Build history of the part. All positions in model axes, mm. Give positions to 0.01 mm unless a question says otherwise; leave off trailing zeros. Write each loop counter-clockwise with the first axis right and the second up, starting at its lowest first coordinate (ties: lowest second). Pieces come first, ordered by that corner, then holes.
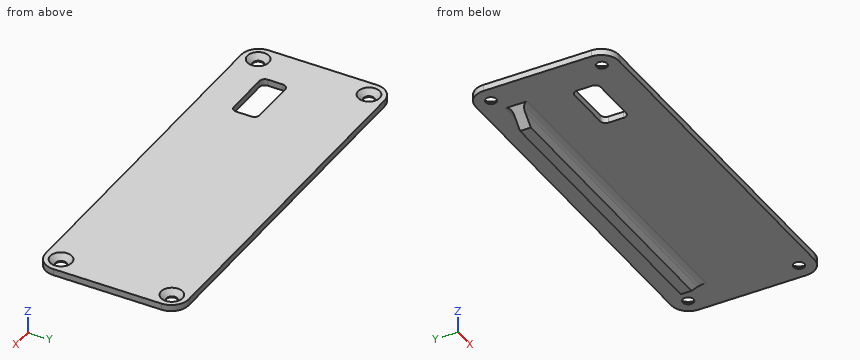
Autodesk Inventor part; units mm, degrees
ref_plane "YZ Plane" through (0, 0, 0) normal (1, 0, 0) x (0, 1, 0)
ref_plane "XZ Plane" through (0, 0, 0) normal (0, 1, 0) x (-1, 0, 0)
ref_plane "XY Plane" through (0, 0, 0) normal (0, 0, 1) x (1, 0, 0)
sketch "Sketch1" plane through (0, 0, 0) normal (0, 0, 1) x (1, 0, 0)
  line L0 (-35.5, 13.25) -> (35.5, 13.25)
  line L1 (35.5, 13.25) -> (35.5, -13.25)
  line L2 (35.5, -13.25) -> (-35.5, -13.25)
  line L3 (-35.5, -13.25) -> (-35.5, 13.25)
  point P0 (0, 0)
  dimension "d0" = 26.5
  dimension "d1" = 71
  dimension "d2" = 35.5
  dimension "d3" = 13.25
extrude "Extrusion1" add sketch "Sketch1" along normal blind 1.2
fillet "Fillet1" radius 3.25 4 edges at (-35.5, 13.25, 0.6) (-35.5, -13.25, 0.6) (35.5, -13.25, 0.6) (35.5, 13.25, 0.6)
sketch "Sketch2" plane through (0, 0, 1.2) normal (0, 0, 1) x (1, 0, 0)
  line L0 (32.25, 13.25) -> (-32.25, 13.25)
  line L1 (-35.5, 10) -> (-35.5, -10)
  line L2 (-32.25, -13.25) -> (32.25, -13.25)
  line L3 (35.5, -10) -> (35.5, 10)
  point P0 (0, 0)
  point P1 (-32.5, 10.25)
  point P2 (32.5, 10.25)
  point P3 (32.5, -10.25)
  point P4 (-32.5, -10.25)
  dimension "d7" = 3
  dimension "d8" = 3
  dimension "d9" = 3
  dimension "d10" = 3
  dimension "d11" = 3
  dimension "d12" = 3
  dimension "d13" = 3
  dimension "d14" = 3
hole "Hole1" at (-32.5, 10.25, 1.2) at (32.5, 10.25, 1.2) at (32.5, -10.25, 1.2) at (-32.5, -10.25, 1.2) direction (0, 0, -1) diameter 2 depth 4 tip angle 118 countersink diameter 4 countersink angle 90
sketch "Sketch3" plane through (0, 0, 1.2) normal (0, 0, 1) x (1, 0, 0)
  line L0 (-28.2, -2.25) -> (-17.8, -2.25)
  line L1 (-17.8, -2.25) -> (-17.8, -7.05)
  line L2 (-17.8, -7.05) -> (-28.2, -7.05)
  line L3 (-28.2, -7.05) -> (-28.2, -2.25)
  line L4 (-35.5, 10) -> (-35.5, -10)
  line L5 (-32.25, -13.25) -> (32.25, -13.25)
  point P0 (0, 0)
  dimension "d22" = 7.3
  dimension "d23" = 17.7
  dimension "d24" = 6.2
  dimension "d25" = 11
extrude "Extrusion2" cut sketch "Sketch3" against normal blind 1.2
fillet "Fillet2" radius 1 4 edges at (-28.2, -2.25, 0.6) (-28.2, -7.05, 0.6) (-17.8, -2.25, 0.6) (-17.8, -7.05, 0.6)
sketch "Sketch4" plane through (0, 0, 0) normal (0, 0, -1) x (-1, 0, 0)
  line L0 (-29.5, 8.25) -> (29.5, 8.25)
  line L1 (29.5, 8.25) -> (29.5, 6.25)
  line L2 (29.5, 6.25) -> (-29.5, 6.25)
  line L3 (-29.5, 6.25) -> (-29.5, 8.25)
  line L4 (-35.5, -10) -> (-35.5, 10)
  line L5 (35.5, 10) -> (35.5, -10)
  line L6 (-32.25, 13.25) -> (32.25, 13.25)
  point P0 (0, 0)
  dimension "d29" = 6
  dimension "d30" = 6
  dimension "d31" = 5
  dimension "d32" = 2
extrude "Extrusion3" add sketch "Sketch4" along normal blind 3
fillet "Fillet3" radius 1 2 edges at (0, 6.25, 0) (0, 8.25, 0)
chamfer "Chamfer1" distance 3 angle 45 2 edges at (29.5, 7.25, -3) (-29.5, 7.25, -3)
properties part number "cover"
(1) Saw through at A-A, the plane y = 2.25. List the corners of the cut face in (x, z).
(2) Drop flat-ended pins along their axis: pin 1 (6 mm diameter, centred on x = -8.5, y = 1.5, fed in from -Z); pin 2 (1.5 mm diameter, centred on y = 5, z = -1.5, fed in from -X); pin 3 (1 mm diameter, centred on x = 4.5, z = -1.5, fed in from +Y); pin 4 (1 mm diameter, centred on x = 13.5, z = -1.5, fed in from -Y). Give the stop position or say it passes through.
(3) Probe line 1 (Y direction, x = 32.5, z = 0.15); line 2 (X direction, y = 10.25, z = 0.1); line 3 (Y direction, x = 21, z = -1.8). List the from-to ranges inside material, lowest first.
Computed values:
1. outline: (-35.5, 0) - (35.5, 0) - (35.5, 1.2) - (-35.5, 1.2) - close
2. pin 1: stops at z = 0
2. pin 2: passes through
2. pin 3: stops at y = 8.25
2. pin 4: stops at y = 6.25
3. line 1: y = -13.24 to -11.25, -9.25 to 9.25, 11.25 to 13.24
3. line 2: x = -35.49 to -33.5, -31.5 to 31.5, 33.5 to 35.49
3. line 3: y = 6.25 to 8.25
